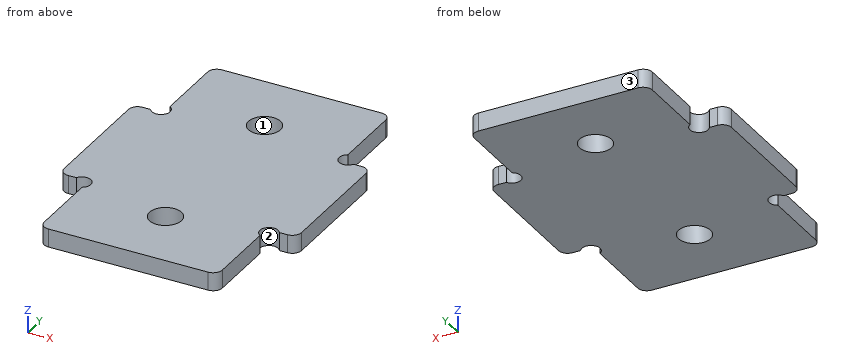
```python
from build123d import *

# Parameters (mm, degrees)
SKETCH_1_W          = 19.5
SKETCH_1_H          = 35
EXTRUDE_1_DEPTH     = 2
SKETCH_3_R          = 1.75
CUT_EXTRUDE_1_DEPTH = 41.115458367
SKETCH_4_W          = 3.25
SKETCH_4_H          = 15
EXTRUDE_2_DEPTH     = 2
SKETCH_5_R          = 1
CUT_EXTRUDE_2_DEPTH = 10
FILLET_1_R          = 1


with BuildPart() as part:
    # 草图1 → 凸台-拉伸1 (new body)
    with BuildSketch(Plane.XY):
        with Locations((9.75, 17.5)):
            Rectangle(SKETCH_1_W, SKETCH_1_H)
    extrude(amount=EXTRUDE_1_DEPTH)

    # 草图3 → 切除-拉伸1 (cut, through all)
    with BuildSketch(Plane.XY.offset(2)):
        with Locations((9.75, 27.5)):
            Circle(SKETCH_3_R)
        with Locations(Location((9.75, 7.5, 0), (0, 0, 180))):
            Circle(SKETCH_3_R)
    extrude(amount=-CUT_EXTRUDE_1_DEPTH, mode=Mode.SUBTRACT)

    # 草图4 → 凸台-拉伸2 (add)
    with BuildSketch(Plane.XY.offset(2)):
        with Locations((21.125, 17.5)):
            Rectangle(SKETCH_4_W, SKETCH_4_H)
        with Locations((-1.625, 17.5)):
            Rectangle(SKETCH_4_W, SKETCH_4_H)
    extrude(amount=-EXTRUDE_2_DEPTH)

    # 草图5 → 切除-拉伸2 (cut)
    with BuildSketch(Plane.XY.offset(2)):
        with Locations((20, 25.5)):
            Circle(SKETCH_5_R)
        with Locations((20, 9.5)):
            Circle(SKETCH_5_R)
        with Locations((-0.5, 9.5)):
            Circle(SKETCH_5_R)
        with Locations((-0.5, 25.5)):
            Circle(SKETCH_5_R)
    extrude(amount=-CUT_EXTRUDE_2_DEPTH, mode=Mode.SUBTRACT)

    # 圆角1
    fillet_1_edges = [part.edges().sort_by_distance(p)[0] for p in [
        (22.75, 10, 1),
        (22.75, 25, 1),
        (-3.25, 10, 1),
        (-3.25, 25, 1),
        (19.5, 35, 1),
        (19.5, 0, 1),
        (0, 0, 1),
        (0, 35, 1),
    ]]
    fillet(fillet_1_edges, radius=FILLET_1_R)


solid = part.part
```
Input: part model. Units: mm. Frame: model coordinates. Face numbers are marked on the shaded views. Give positions to 0.01 mm unless a question says otherwise; leave off trailing zeros. Loops run counter-clockwise (first coordinate to the right, second up) from the corner with the lowest first, then second, coordinate; pieces in that order, holes last. Notation, with made-up numbers: (-2, 48) -> (5, 48) arc R9 cw to (5, 61) -> close; hole circle Ø9 at (8.25, -26.5). An arc over 180 degrees is marked (long way). Use a Markdown table: item, result.
Q1. Section query C-C, the plane x = 8.5. Return the cut outline in (y, z), plus the area to 3 significant figures.
Entries:
| item | result |
|---|---|
| outline | (0, 0) -> (6.28, 0) -> (6.28, 2) -> (0, 2) -> close; (8.72, 0) -> (26.28, 0) -> (26.28, 2) -> (8.72, 2) -> close; (28.72, 0) -> (35, 0) -> (35, 2) -> (28.72, 2) -> close |
| area | 60.2 mm² |
Q2. First-contact query: P1, Ø1, axis at y = 3.5, z = 1, coming from the -X side; P2, Ø1, axis at y = 32, z = 1, coming from the +X side; P3, Ø0.7, axis at x = -1.5, z = 0.5, coming from the -Y side. Flat tips, straight axial feed; report the tip coordinate or a pass-through.
Entries:
| item | result |
|---|---|
| P1 | stops at x = 0 |
| P2 | stops at x = 19.5 |
| P3 | stops at y = 10 |
Q3. Ray query, probe 1 along Y at (x, z) = (9.75, 1.15); probe 2 along Y at (x, z) = (8.25, 1.25); probe 3 along X at (y, z) = (25.5, 1.2). Return the intervals inside material, ascending. Write a range as from..to.
Entries:
| item | result |
|---|---|
| probe 1 | y = 0..5.75, 9.25..25.75, 29.25..35 |
| probe 2 | y = 0..6.6, 8.4..26.6, 28.4..35 |
| probe 3 | x = 0.5..19 |
Q4. Section query D-D, the plane x = -0.5. Return the cut outline in (y, z).
Entries:
| item | result |
|---|---|
| outline | (10.5, 0) -> (24.5, 0) -> (24.5, 2) -> (10.5, 2) -> close |
Q5. Section query B-B, the plane y = 27.5. Return the cut outline in (x, z).
Entries:
| item | result |
|---|---|
| outline | (0, 0) -> (8, 0) -> (8, 2) -> (0, 2) -> close; (11.5, 0) -> (19.5, 0) -> (19.5, 2) -> (11.5, 2) -> close |
Q6. Section query A-A, the plane z = 1.55. Return the cut outline in (x, y).
Entries:
| item | result |
|---|---|
| outline | (-3.25, 11) arc R1 ccw to (-2.25, 10) -> (-1.37, 10) arc R1 cw (long way) to (0, 8.63) -> (0, 1) arc R1 ccw to (1, 0) -> (18.5, 0) arc R1 ccw to (19.5, 1) -> (19.5, 8.63) arc R1 cw (long way) to (20.87, 10) -> (21.75, 10) arc R1 ccw to (22.75, 11) -> (22.75, 24) arc R1 ccw to (21.75, 25) -> (20.87, 25) arc R1 cw (long way) to (19.5, 26.37) -> (19.5, 34) arc R1 ccw to (18.5, 35) -> (1, 35) arc R1 ccw to (0, 34) -> (0, 26.37) arc R1 cw (long way) to (-1.37, 25) -> (-2.25, 25) arc R1 ccw to (-3.25, 24) -> close; hole circle Ø3.5 at (9.75, 7.5); hole circle Ø3.5 at (9.75, 27.5) |
Q7. Pull-direction query (X, two-part tool) for the marked faces 1, 2 and 3; classes: pulls with the +X half, pulls with the -X half, needs draft (parallel to the pull), parting line crosses it, or undercut.
Entries:
| item | result |
|---|---|
| face 1 | undercut |
| face 2 | undercut |
| face 3 | needs draft |
